Could you check a few things on this drawing? It's one solid part, dimensions in mm from its lowest x, y, z. Coordinates: 2 decimals unless noted, no trailing zeros. Loops run counter-clockwise (first coordinate to the right, second up) from the corner with the lowest first, then second, coordinate; pieces in that order, holes last.
1) Imagine slicing it at C-C on z = 7. Please give me the cut outline in (x, y).
2) If I drill on line 1 along Y through (x, z) = (25, 15.5); line 2 along X through (y, z) = (19, 18.5); line 3 along X through (y, z) = (16, 10.25), over which ranges is the centre line in solid material (lowest first)?
3) Imagine slicing it at A-A on x = 25. Please give me the cut outline in (y, z), plus the area to 3 significant figures.
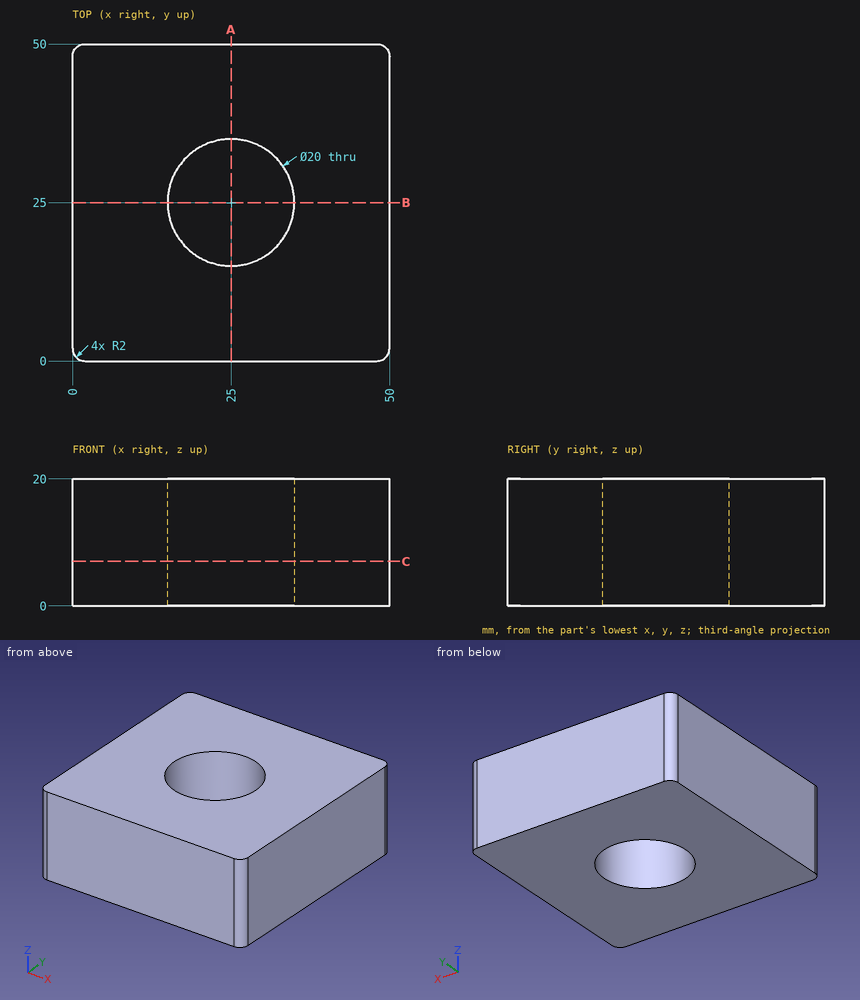
Filled in:
1. outline: (0, 2) arc R2 ccw to (2, 0) - (48, 0) arc R2 ccw to (50, 2) - (50, 48) arc R2 ccw to (48, 50) - (2, 50) arc R2 ccw to (0, 48) - close; hole circle Ø20 at (25, 25)
2. line 1: y = 0 to 15, 35 to 50
2. line 2: x = 0 to 17, 33 to 50
2. line 3: x = 0 to 20.64, 29.36 to 50
3. outline: (0, 0) - (15, 0) - (15, 20) - (0, 20) - close; (35, 0) - (50, 0) - (50, 20) - (35, 20) - close
3. area: 600 mm2
